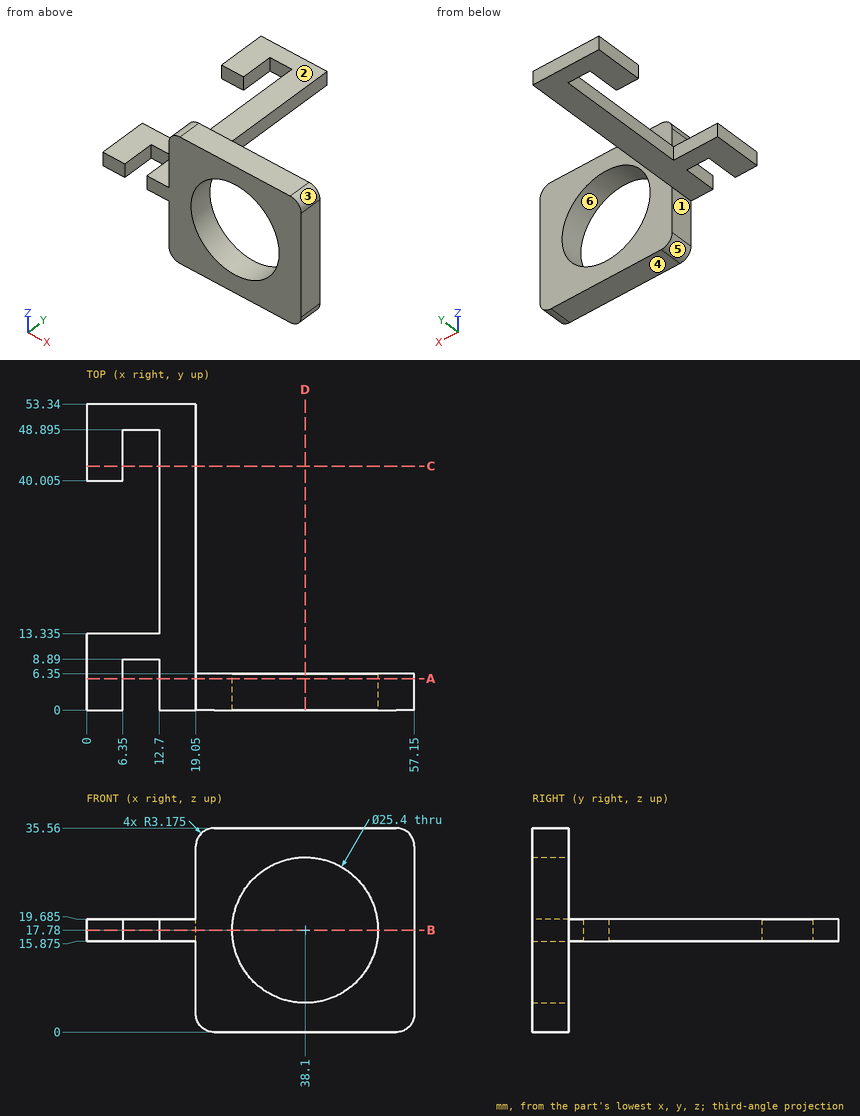
Could you check a few things on this drawing? It's one solid part, dimensions in mm from its lowest x, y, z. A direction names the side the tool comes from. Coordinates: 2 decimals unless noted, no trailing zeros. Order: outer loops, then holes, each group sorted by start corner. A loop starts at its lowest first (then second) coordinate and runs counter-clockwise, first axis right, second up. Notation, with made-up numbers: (23.5, 50.5) - (55.5, 50.5) arc R15 ccw to (55.5, 78.5) - close; hole circle Ø2 at (-8, 84). An arc over 180 degrees is marked (long way). Answer as a JSON object with one key per item and string values. Group by question number.
Q1. On a 3-axis mill with a long thin cutter (end or side, diameter ignored), from which of +Z, -Z, +X, -X, +Y, -Y can I reach the whole of each face in a straight line? I mean the marked faces 1, 2 and 3. Say none if no direction works.
Q2. Imagine slicing it at C-C (y = 42.5). Please give me the cut outline in (x, z) (3 decimals), and give its area (3 significant figures).
Q3. Imagine slicing it at B-B (z = 17.78). Please give me the cut outline in (x, y) (3 decimals), and give its area (3 significant figures).
Q4. We'd pull the mould along X, two halves only. Please class the marked faces 4, 5 and 6: +X half, -X half, draft (parallel to the pull), parting line (faces both ways), or undercut.
Q5. Imagine slicing it at D-D (x = 38.1). Please give me the cut outline in (y, z), and give its area (3 significant figures).
Q6. I need wall thicknesses on line 1 (X direction, y = 2.25, z = 17.78); line 2 (Z direction, x = 38.1, y = 3.75); line 3 (Y direction, x = 55.5, z = 3). Which ranges of each line are inside material? Lowest first, please. Write a range as from..to.
Q7. Imagine slicing it at A-A (y = 5.5). Please give me the cut outline in (x, z) (3 decimals), and give its area (3 significant figures).
Q8. Will these pins go through, and if not, where does the flat tip stop? P1, Ø10, axis at y = 9.5, z = 9, coming from the -X side; P2, Ø5, axis at x = 14.5, y = 42, coming from the -Z side (3 decimals); P3, Ø4, axis at x = 9, z = 18.5, coming from the -Y side.
Determined:
{
 "1": {"face 1": "-Z, -X, +Y, -Y", "face 2": "+Z, -X, +Y, -Y", "face 3": "+Z, +X, +Y, -Y"},
 "2": {"outline": "(0, 15.875) - (6.35, 15.875) - (6.35, 19.685) - (0, 19.685) - close; (12.7, 15.875) - (19.05, 15.875) - (19.05, 19.685) - (12.7, 19.685) - close", "area": "48.4 mm2"},
 "3": {"outline": "(0, 0) - (6.35, 0) - (6.35, 8.89) - (12.7, 8.89) - (12.7, 0) - (25.4, 0) - (25.4, 6.35) - (19.05, 6.35) - (19.05, 53.34) - (0, 53.34) - (0, 40.005) - (6.35, 40.005) - (6.35, 48.895) - (12.7, 48.895) - (12.7, 13.335) - (0, 13.335) - close; (50.8, 0) - (57.15, 0) - (57.15, 6.35) - (50.8, 6.35) - close", "area": "645 mm2"},
 "4": {"face 4": "draft", "face 5": "-X half", "face 6": "undercut"},
 "5": {"outline": "(0, 0) - (6.35, 0) - (6.35, 5.08) - (0, 5.08) - close; (0, 30.48) - (6.35, 30.48) - (6.35, 35.56) - (0, 35.56) - close", "area": "64.5 mm2"},
 "6": {"line 1": "x = 0..6.35, 12.7..25.4, 50.8..57.15", "line 2": "z = 0..5.08, 30.48..35.56", "line 3": "y = 0..6.35"},
 "7": {"outline": "(0, 15.875) - (6.35, 15.875) - (6.35, 19.685) - (0, 19.685) - close; (12.7, 15.875) - (19.05, 15.875) - (19.05, 3.175) arc R3.175 ccw to (22.225, 0) - (53.975, 0) arc R3.175 ccw to (57.15, 3.175) - (57.15, 32.385) arc R3.175 ccw to (53.975, 35.56) - (22.225, 35.56) arc R3.175 ccw to (19.05, 32.385) - (19.05, 19.685) - (12.7, 19.685) - close; hole circle Ø25.4 at (38.1, 17.78)", "area": "888 mm2"},
 "8": {"P1": "stops at x = 19.05", "P2": "stops at z = 15.875", "P3": "stops at y = 8.89"}
}
